Could you check a few things on this drawing? It's one solid part, dimensions in mm from its lowest x, y, z. A direction names the side the tool comes from. Give positions to 0.01 mm unless a question says otherwise; leave off trailing zeros. Loops run counter-clockwise (first coordinate to the right, second up) from the corner with the lowest first, then second, coordinate; pieces in that order, holes last. Notation, with made-up numbers: (27.5, 75) -> (60.5, 75) arc R20 cw to (60.5, 107) -> close; hole circle Ø6 at (6, 84). An arc over 180 degrees is marked (long way). Use CSV: the item, a comma, the result in double quotes.
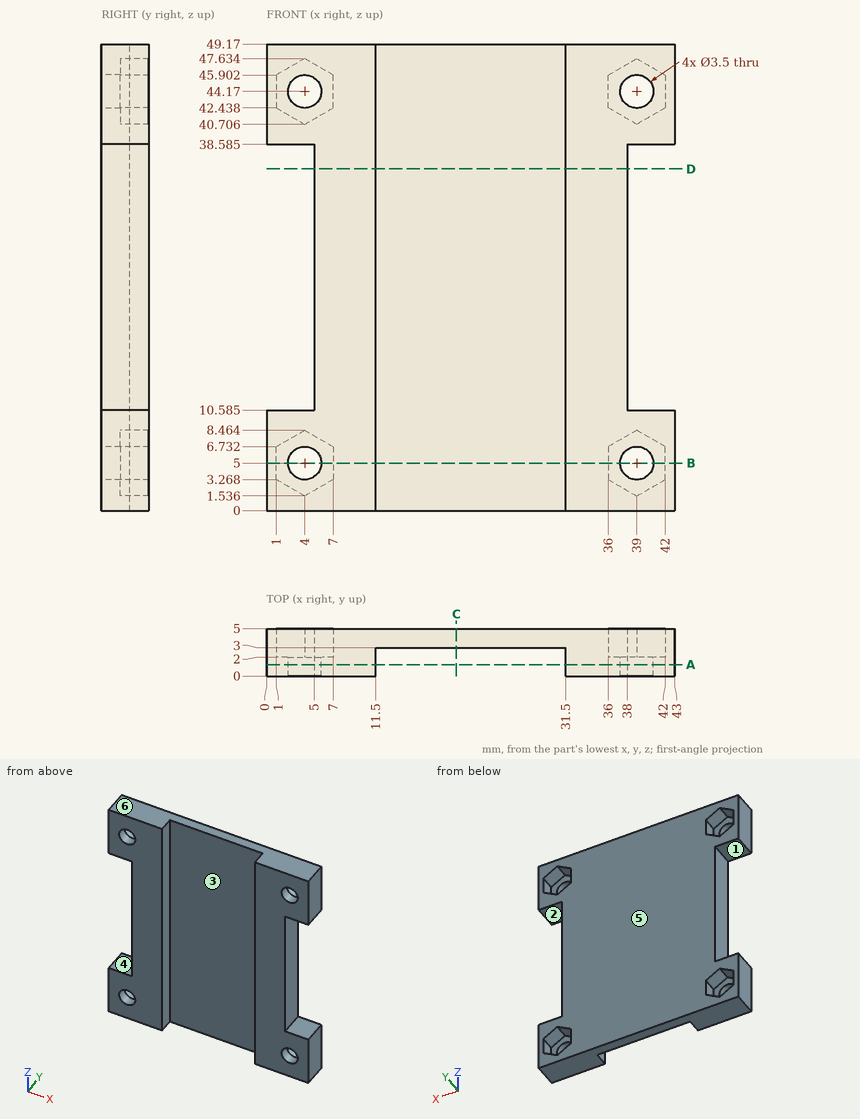
(1) If we section it at B-B, the plane z = 5: Write out the boundary of the cut face in (x, y), then the cut area to 3 significant figures.
Answer sheet:
outline,"(0, 0) -> (2.25, 0) -> (2.25, 2) -> (1, 2) -> (1, 5) -> (0, 5) -> close; (5.75, 0) -> (11.5, 0) -> (11.5, 3) -> (31.5, 3) -> (31.5, 0) -> (37.25, 0) -> (37.25, 2) -> (36, 2) -> (36, 5) -> (7, 5) -> (7, 2) -> (5.75, 2) -> close; (40.75, 0) -> (43, 0) -> (43, 5) -> (42, 5) -> (42, 2) -> (40.75, 2) -> close"
area,"105 mm2"
(2) Will these pins go through, and if not, where does the flat tip stop? pin 1 Ø1.8 at (x, z) = (38, 6) entering from +Y; pin 2 Ø2.5 at (y, z) = (2, 30.5) entering from +X; pin 3 Ø6 at (x, z) = (24.5, 20.5) entering from -Y; pin 4 Ø3 at (x, z) = (39, 5) entering from -Y.
Answer sheet:
pin 1,"stops at y = 2"
pin 2,"stops at x = 38"
pin 3,"stops at y = 3"
pin 4,"passes through"
(3) Which directions (+Z, -Z, +X, -X, +Y, -Y) give clear straight access to the entire face, cutting with the end or side of a thin tool? Please do the marked faces 1, 2 and 3.
Answer sheet:
face 1,"-X, +Y, -Y"
face 2,"+X, +Y, -Y"
face 3,"+Z, -Z, -Y"
(4) If we section it at D-D, the plane z = 36: Write out the boundary of the cut face in (x, y), then the cut area to 3 significant figures.
Answer sheet:
outline,"(5, 0) -> (11.5, 0) -> (11.5, 3) -> (31.5, 3) -> (31.5, 0) -> (38, 0) -> (38, 5) -> (5, 5) -> close"
area,"105 mm2"
(5) We'd pull the mould along Z, two halves only. Please class the marked faces 4, 5 and 6: released by +Z, released by -Z, zero draft, split by the parting line, or undercut.
Answer sheet:
face 4,"undercut"
face 5,"zero draft"
face 6,"released by +Z"
(6) If I drill on L1, parallel to X at y = 1.1, z = 44.17; L2, parallel to X at y = 0.9, z = 27.5; L3, parallel to X at y = 2.1, z = 3 (1 decimal), over which ranges is the centre line in solid material (lowest first)? Write a range as from..to.
Answer sheet:
L1,"x = 0..2.25, 5.75..11.5, 31.5..37.25, 40.75..43"
L2,"x = 5..11.5, 31.5..38"
L3,"x = 0..1.5, 6.5..11.5, 31.5..36.5, 41.5..43"
(7) If we section it at A-A, the plane y = 1.2: Write out the boundary of the cut face in (x, z) (3 decimals), then the cut area to 3 significant figures.
Answer sheet:
outline,"(0, 0) -> (11.5, 0) -> (11.5, 49.17) -> (0, 49.17) -> (0, 38.585) -> (5, 38.585) -> (5, 10.585) -> (0, 10.585) -> close; (31.5, 0) -> (43, 0) -> (43, 10.585) -> (38, 10.585) -> (38, 38.585) -> (43, 38.585) -> (43, 49.17) -> (31.5, 49.17) -> close; hole circle Ø3.5 at (4, 5); hole circle Ø3.5 at (4, 44.17); hole circle Ø3.5 at (39, 5); hole circle Ø3.5 at (39, 44.17)"
area,"812 mm2"
(8) If we section it at C-C, the plane x = 20: Write out the boundary of the cut face in (y, z).
Answer sheet:
outline,"(3, 0) -> (5, 0) -> (5, 49.17) -> (3, 49.17) -> close"
